from build123d import *

# Parameters (mm, degrees)
SKETCH1_R           = 3.5
BOSS_EXTRUDE1_DEPTH = 2
CHAMFER1_SIZE       = 1
SKETCH2_R           = 1.5
CUT_EXTRUDE1_DEPTH  = 2


with BuildPart() as part:
    # Sketch1 → Boss-Extrude1 (new body)
    with BuildSketch(Plane(origin=(0, 0, 0), x_dir=(1, 0, 0), z_dir=(0, 1, 0))):
        Circle(SKETCH1_R)
    extrude(amount=BOSS_EXTRUDE1_DEPTH)

    # Chamfer1
    chamfer1_edges = [part.edges().sort_by_distance(p)[0] for p in [
        (-3.5, 2, 0),
    ]]
    chamfer(chamfer1_edges, length=CHAMFER1_SIZE)

    # Sketch2 → Cut-Extrude1 (cut)
    with BuildSketch(Plane(origin=(0, 2, 0), x_dir=(1, 0, 0), z_dir=(0, 1, 0))):
        Circle(SKETCH2_R)
    extrude(amount=-CUT_EXTRUDE1_DEPTH, mode=Mode.SUBTRACT)


solid = part.part
Geometry check sheet. Reference: the model listing, model coordinates, mm. Round coordinates to 2 decimals unless told otherwise and drop trailing zeros. Order: outer loops, then holes, each group sorted by start corner. A loop starts at its lowest first (then second) coordinate and runs counter-clockwise, first axis right, second up. Notation, with made-up numbers: M -5.75,-24.75 L 18.25,-24.75 A16 cw 18.25,-20.75 Z; hole C 5,55 d8. An arc over 180 degrees is marked long. Write each question's results on one line, items separated by ' | '. Start each with the question number.
1. Go/stop test with a flat-tipped pin: P1, Ø1, axis at x = -1.5, z = -1, coming from the -Y side. Record where the tip stops, or that it passes through.
2. Cross-section at A-A on z = 0. Record the boundary of the cut face in (x, y).
3. Draft check along X on faces 1 (the face through (3.233, 0.493, 1.341)), 2 (the face through (0, 0, 2)), 3 (the face through (-1.5, 1.01, -0.07)). Enter one of: pulls with the +X half, pulls with the -X half, needs draft (parallel to the pull), parting line crosses it, or undercut.
4. Material ranges on L1, parallel to X at y = 0.95, z = 0; L2, parallel to Z at x = 0, y = 1.7; L3, parallel to Z at x = 1, y = 0.5, recorded low to high. Write a range as from..to.
5. Cross-section at B-B on x = 0. Record the boundary of the cut face in (y, z), plus the area to 3 significant figures.
6. Cross-section at C-C on y = 1.6. Record the boundary of the cut face in (x, z), plus the area to 3 significant figures.
Resolved:
1) P1: y = 0
2) outline: M -3.5,0 L -1.5,0 L -1.5,2 L -2.5,2 L -3.5,1 Z; M 1.5,0 L 3.5,0 L 3.5,1 L 2.5,2 L 1.5,2 Z
3) face 1: parting line crosses it | face 2: needs draft | face 3: undercut
4) L1: -3.5..-1.5, 1.5..3.5 | L2: -2.8..-1.5, 1.5..2.8 | L3: -3.35..-1.12, 1.12..3.35
5) outline: M 0,-3.5 L 1,-3.5 L 2,-2.5 L 2,-1.5 L 0,-1.5 Z; M 0,1.5 L 2,1.5 L 2,2.5 L 1,3.5 L 0,3.5 Z | area: 7.00 mm2
6) outline: C 0,0 d5.8; hole C 0,0 d3 | area: 19.4 mm2
